Work out the finished part from the listing and answer in its coordinate system (mm). Face numbers are marked on the shaded views. A direction names the side the tool comes from. Coordinates: 2 decimals unless noted, no trailing zeros. Order: outer loops, then holes, each group sorted by start corner. A loop starts at its lowest first (then second) coordinate and runs counter-clockwise, first axis right, second up. Notation, with made-up numbers: (26, -22) -> (51, -22) arc R25 cw to (51, -4) -> close; hole circle Ø11 at (7.5, -8.5). An arc over 180 degrees is marked (long way). Answer as CSV lines item,"result". Start each with the question number.
Item 1: Straight lines are drawn through the part: L1, parallel to X at y = 11.5, z = -12; L2, parallel to X at y = 5.25, z = 4; L3, parallel to X at y = 11.8, z = 0. For each, find the intervals that lie inside material, in ascending order.
Item 2: Section C-C (z = 0) is taken. Write down the section's boundary in (x, y).
Item 3: Which of the six approach directions +Z, -Z, +X, -X, +Y, -Y give full straight-line access (tool end or side, diameter ignored) to the marked faces 1 and 2?
Item 4: Section A-A (x = 38.5) is taken. Write down the section's boundary in (y, z), then the cut area to 4 significant figures.
Item 5: Section B-B (x = 11) is taken. Write down the section's boundary in (y, z), then the cut area to 3 significant figures.
Item 6: Section D-D (y = 4.25) is taken. Write down the section's boundary in (x, z), then the cut area to 3 significant figures.
Item 7: For a pull along Z with two mould halves and no side action, classify the marked faces 3, 4 and 5 as pulls with the +Z half, pulls with the -Z half, needs draft (parallel to the pull), parting line crosses it, or undercut.
Item 8: Each of these flat-tipped pins is pushed along its axis until it touches: pin 1 Ø3 at (x, z) = (-17.5, 9) entering from -Y; pin 2 Ø12 at (x, z) = (12.5, -10) entering from +Y. Where does it stop, or does it pass through?
```python
from build123d import *

# Parameters (mm, degrees)
SKETCH_1_W          = 115
SKETCH_1_H          = 50
EXTRUDE_1_DEPTH     = 13
SKETCH_2_W          = 113
SKETCH_2_H          = 48
CUT_EXTRUDE_1_DEPTH = 10
SKETCH_3_R          = 8.25
SKETCH_3_R_2        = 11.25
SKETCH_3_R_3        = 6
SKETCH_3_W          = 26.7
SKETCH_3_H          = 12
SKETCH_3_W_2        = 2.2
SKETCH_3_H_2        = 5.2
CUT_EXTRUDE_2_DEPTH = 10


with BuildPart() as part:
    # 草图1 → 凸台-拉伸1 (new body)
    with BuildSketch(Plane(origin=(0, 0, 0), x_dir=(1, 0, 0), z_dir=(0, 1, 0))):
        Rectangle(SKETCH_1_W, SKETCH_1_H)
    extrude(amount=EXTRUDE_1_DEPTH)

    # 草图2 → 切除-拉伸1 (cut)
    with BuildSketch(Plane.XZ):
        Rectangle(SKETCH_2_W, SKETCH_2_H)
    extrude(amount=-CUT_EXTRUDE_1_DEPTH, mode=Mode.SUBTRACT)

    # 草图3 → 切除-拉伸2 (cut)
    with BuildSketch(Plane(origin=(0, 13, 0), x_dir=(1, 0, 0), z_dir=(0, 1, 0))):
        with Locations(Location((-39.5, 0, 0), (0, 0, 270))):
            Circle(SKETCH_3_R)
        with Locations(Location((38.5, 0, 0), (0, 0, 270))):
            Circle(SKETCH_3_R_2)
        with Locations(Location((-14, 12, 0), (0, 0, 270))):
            Circle(SKETCH_3_R)
        with Locations(Location((11, 12, 0), (0, 0, 270))):
            Circle(SKETCH_3_R_3)
        with Locations((0, -17.039877017)):
            Rectangle(SKETCH_3_W, SKETCH_3_H)
        with Locations((-15, -5)):
            Rectangle(SKETCH_3_W_2, SKETCH_3_H_2)
        with Locations((15, -5)):
            Rectangle(SKETCH_3_W_2, SKETCH_3_H_2)
        with Locations((5, -5)):
            Rectangle(SKETCH_3_W_2, SKETCH_3_H_2)
        with Locations((-5, -5)):
            Rectangle(SKETCH_3_W_2, SKETCH_3_H_2)
    extrude(amount=-CUT_EXTRUDE_2_DEPTH, mode=Mode.SUBTRACT)


solid = part.part
```
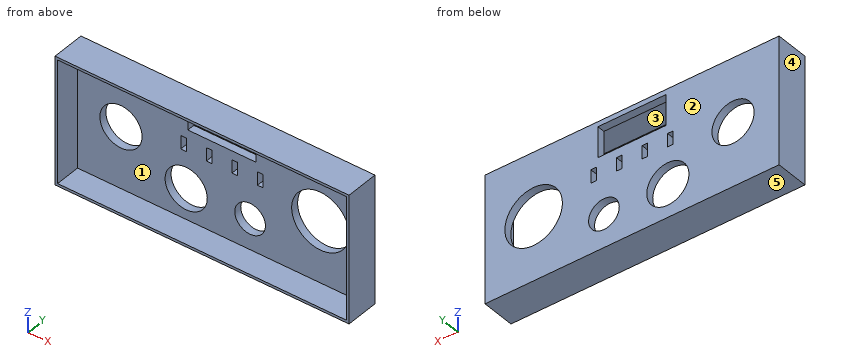
Checked values:
1,L1,"x = -57.5 to -22.25, -5.75 to 5, 17 to 57.5"
1,L2,"x = -57.5 to -56.5, 56.5 to 57.5"
1,L3,"x = -57.5 to -47.75, -31.25 to 27.25, 49.75 to 57.5"
2,outline,"(-57.5, 0) -> (-56.5, 0) -> (-56.5, 10) -> (-47.75, 10) -> (-47.75, 13) -> (-57.5, 13) -> close; (-31.25, 10) -> (27.25, 10) -> (27.25, 13) -> (-31.25, 13) -> close; (49.75, 10) -> (56.5, 10) -> (56.5, 0) -> (57.5, 0) -> (57.5, 13) -> (49.75, 13) -> close"
3,face 1,"-Y"
3,face 2,"+Z, -Z, +X, -X, +Y"
4,outline,"(0, -25) -> (13, -25) -> (13, -11.25) -> (10, -11.25) -> (10, -24) -> (0, -24) -> close; (0, 24) -> (10, 24) -> (10, 11.25) -> (13, 11.25) -> (13, 25) -> (0, 25) -> close"
4,area,"102.5 mm^2"
5,outline,"(0, -25) -> (13, -25) -> (13, -18) -> (10, -18) -> (10, -24) -> (0, -24) -> close; (0, 24) -> (10, 24) -> (10, 23.04) -> (13, 23.04) -> (13, 25) -> (0, 25) -> close; (10, -6) -> (13, -6) -> (13, 11.04) -> (10, 11.04) -> close"
5,area,"98.0 mm^2"
6,outline,"(-57.5, -25) -> (57.5, -25) -> (57.5, 25) -> (-57.5, 25) -> close; hole (-56.5, -24) -> (56.5, -24) -> (56.5, 24) -> (-56.5, 24) -> close"
6,area,"326 mm^2"
7,face 3,"undercut"
7,face 4,"needs draft"
7,face 5,"pulls with the -Z half"
8,pin 1,"stops at y = 10"
8,pin 2,"stops at y = 13"
